Autodesk Inventor part; units mm, degrees
ref_plane "YZ Plane" through (0, 0, 0) normal (1, 0, 0) x (0, 1, 0)
ref_plane "XZ Plane" through (0, 0, 0) normal (0, 1, 0) x (-1, 0, 0)
ref_plane "XY Plane" through (0, 0, 0) normal (0, 0, 1) x (1, 0, 0)
sketch "Sketch1" plane through (0, 0, 0) normal (0, 1, 0) x (-1, 0, 0)
  line L0 (15, 20) -> (-15, 20)
  line L1 (-15, 20) -> (-15, -20)
  line L2 (-15, -20) -> (15, -20)
  line L3 (15, -20) -> (15, 20)
  line L4 (15, 20) -> (-15, -20) construction
  line L5 (-15, 20) -> (15, -20) construction
  line L6 (21, 0) -> (-21, 0) construction
  line L7 (0, -28) -> (0, 28) construction
  line L8 (6, 0) -> (0, 0) construction
  line L9 (6, 3.4) -> (0, 3.4)
  line L10 (0, -3.4) -> (6, -3.4)
  arc A0 (6, -3.4) -> (6, 3.4) centre (6, 0) ccw
  arc A1 (0, 3.4) -> (0, -3.4) centre (0, 0) ccw
  line L11 (-15, 12.5) -> (15, 12.5)
  line L12 (-15, -12.5) -> (15, -12.5)
  point P0 (0, 0)
  point P1 (3, 0)
  point P2 (3, 0)
  point P3 (15, -12.5)
  dimension "d0" = 40
  dimension "d1" = 30
  dimension "d2" = 6
  dimension "d3" = 6.8
  dimension "d19" = 3
  dimension "d35" = 25
extrude "Extrusion1" add sketch "Sketch1" against normal blind 25 contours L3 L11 L1 L0 | L3 L12 L1 L11 | L3 L2 L1 L12 | A0 L10 A1 L9
extrude "Extrusion2" cut sketch "Sketch1" against normal blind 8
sketch "Sketch3" plane through (0, -25, 0) normal (0, -1, 0) x (1, 0, 0)
  circle A0 centre (0, 0) radius 7.5
  dimension "d29" = 15
extrude "Extrusion5" cut sketch "Sketch3" against normal blind 12
extrude "Extrusion6" cut sketch "Sketch1" against normal blind 20 contours L3 L11 L1 L0 | L3 L2 L1 L12
hole "Hole1" at (-3, 0, 0) direction (0, -1, 0) diameter 4.917 depth 13 countersink diameter 6 countersink angle 90
fillet "Fillet1" radius 5 4 edges at (-15, -22.5, 20) (-15, -22.5, -20) (15, -22.5, -20) (15, -22.5, 20)
chamfer "Chamfer1" distance 0.5 angle 45 13 edges at (0, -25, 20) (-13.5355, -25, 18.5355) (-15, -25, 0) (-13.5355, -25, -18.5355) (0, -25, -20) (13.5355, -25, -18.5355) (15, -25, 0) (13.5355, -25, 18.5355) (-7.5, -25, 0) (-15, -14, 12.5) (-15, -14, -12.5) (15, -14, -12.5) (15, -14, 12.5)
equation "\"d4\" = slotTabH + sheetT"
equation "\"d6\" = slotTabH"
equation "\"slotTabH\" = 8"
equation "\"sheetT\" = 17"
equation "\"totalHeight\" = slotTabH + sheetT"
properties part number "TCSM1-X-003" material "Steel"
The model under review builds one solid part; all positions refer to its coordinate system, in mm. A direction names the side the tool comes from. Round coordinates to 2 decimals unless told otherwise and drop trailing zeros. Write each loop counter-clockwise with the first axis right and the second up, starting at its lowest first coordinate (ties: lowest second). Pieces come first, ordered by that corner, then holes. Notation, with made-up numbers: M 56,-35 L 78,-35 A29 cw 78,-8 Z; hole C 13.5,4 d8. An arc over 180 degrees is marked long. Use a Markdown table: item, result. Add a question column.
Q1. We need section A-A, the plane y = -19.5. State the section outline as (x, z) points, plus the area to 3 significant figures.
Q2. We need section B-B, the plane x = 9. State the section outline as (y, z) points.
Q3. Insertion check: pin 1 (2.5 mm diameter, centred on x = -1.5, z = 17.5, fed in from +Y); pin 2 (8 mm diameter, centred on x = -4.5, y = -13.5, fed in from -Z); pin 3 (6 mm diameter, centred on x = 3, y = -13, fed in from +Z). Each pin has a flat end and moves straight along its axis. Give the tip position at first contact, or say it passes through.
Q4. To check wall thickness, follow line 1 (Z direction, x = 0, y = -16.75); line 2 (Z direction, x = -3, y = -7); line 3 (X direction, y = -10, z = 0). State the ranges of each line that lie inside material, in increasing order.
Q5. Machinability: for faces 1 (the face through (-3, -4, 3.4)), 2 (the face through (13.319, -24.858, -18.246)), 3 (the face through (-7.493, -18.83, 0.33)), 4 (the face through (0, -14, -12.5)), 5 (the face through (-13.319, -24.858, 18.246)), which of the approach directions +Z, -Z, +X, -X, +Y, -Y give a long, thin tool a straight path to every point of the face, cutting with its end or side? Answer none if there is none.
Q6. We need section C-C, the plane z = 0. State the section outline as (x, y) points.
Q7. We need section D-D, the plane z = -14. State the section outline as (x, y) points, plus the area to 3 significant figures.
Q8. The part is to be moulded in two halves that separate along X. For faces 6 (the face through (0, -13, 0)), 7 (the face through (13.246, -24.858, 18.319)), 8 (the face through (-9.4, -3.9, -0.1)), 9 (the face through (-3, -4, -3.4)), say which applies: pulls with the +X half, pulls with the -X half, needs draft (parallel to the pull), parting line crosses it, or undercut.
Findings below:
| question | item | result |
|---|---|---|
| 1 | outline | M -15,-12 L -14.5,-12.5 L 14.5,-12.5 L 15,-12 L 15,12 L 14.5,12.5 L -14.5,12.5 L -15,12 Z; hole C 0,0 d15 |
| 1 | area | 573 mm² |
| 2 | outline | M -25,-19.5 L -24.5,-20 L -20,-20 L -20,-12.5 L -8,-12.5 L -8,12.5 L -20,12.5 L -20,20 L -24.5,20 L -25,19.5 Z |
| 3 | pin 1 | stops at y = -20 |
| 3 | pin 2 | stops at z = -12.5 |
| 3 | pin 3 | stops at z = 12.5 |
| 4 | line 1 | z = -12.5 to -7.5, 7.5 to 12.5 |
| 4 | line 2 | z = -3.4 to -2.46, 2.46 to 3.4 |
| 4 | line 3 | x = -15 to -5.46, -0.54 to 15 |
| 5 | face 1 | +Z, +X, -X, +Y |
| 5 | face 2 | -Z, +X, -Y |
| 5 | face 3 | -Y |
| 5 | face 4 | -Z, +X, -X, +Y |
| 5 | face 5 | +Z, -X, -Y |
| 6 | outline | M -15,-24.5 L -14.5,-25 L -8,-25 L -7.5,-24.5 L -7.5,-13 L -5.46,-13 L -5.46,-0.54 L -6,0 L -9.4,0 L -9.4,-8 L -15,-8 Z; M -0.54,-13 L 7.5,-13 L 7.5,-24.5 L 8,-25 L 14.5,-25 L 15,-24.5 L 15,-8 L 3.4,-8 L 3.4,0 L 0,0 L -0.54,-0.54 Z |
| 7 | outline | M -15,-24.5 L -14.5,-25 L 14.5,-25 L 15,-24.5 L 15,-20 L -15,-20 Z |
| 7 | area | 150 mm² |
| 8 | face 6 | undercut |
| 8 | face 7 | pulls with the +X half |
| 8 | face 8 | pulls with the -X half |
| 8 | face 9 | needs draft |
